Answer from the drawing. Dimensions are ordinates in mm from the lowest x, y and z of the part. Coordinates: 2 decimals unless noted, no trailing zeros. Write each loop counter-clockwise with the first axis right and the second up, starting at its lowest first coordinate (ties: lowest second). Pieces come first, ordered by that corner, then holes.
(1) The part is cut by section A-A, the plane x = 40.5. Determine the outline of the cut face in (y, z).
(2) The part is cut by section C-C, the plane y = 99.5. Determine the outline of the cut face in (x, z).
(3) The part is cut by section D-D, the plane x = 23. Determine the outline of the cut face in (y, z), and give its area (3 significant figures).
(4) Given pin 1 (1.2 mm diameter, centred on y = 154.5, z = 1, fed in from -X); pin 2 (2 mm diameter, centred on x = 26.5, z = 1.5, fed in from +Y), each flat-ended and moving along its own axis, determine where each tip first touches the part or whether it passes through.
(5) The part is cut by section B-B, the plane y = 30.5. Determine the outline of the cut face in (x, z).
(6) Straight lines are drawn through the part: line 1 along X through (y, z) = (16, 3.7); line 2 along Y through (x, z) = (65.5, 3.8); line 3 along Y through (x, z) = (86.5, 2.5). For each, find the intervals that lie inside material, in ascending order.
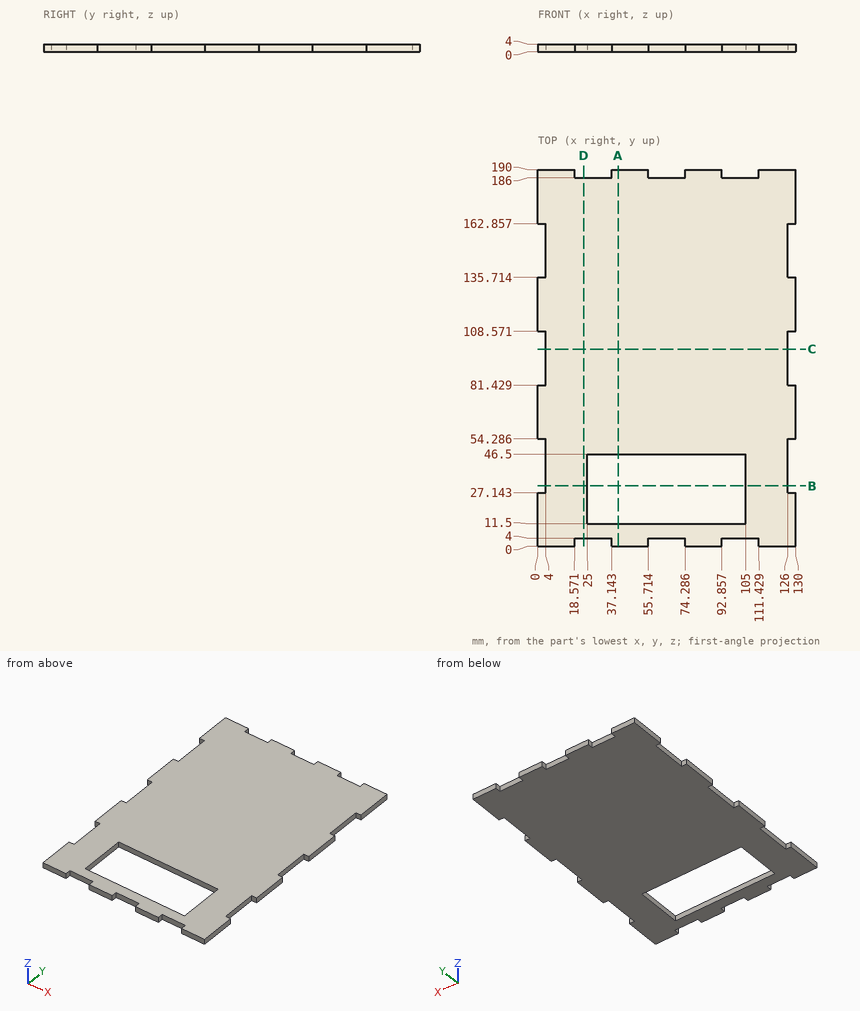
Computed:
1. outline: (0, 0) - (11.5, 0) - (11.5, 4) - (0, 4) - close; (46.5, 0) - (190, 0) - (190, 4) - (46.5, 4) - close
2. outline: (4, 0) - (126, 0) - (126, 4) - (4, 4) - close
3. outline: (4, 0) - (186, 0) - (186, 4) - (4, 4) - close
3. area: 728 mm2
4. pin 1: stops at x = 4
4. pin 2: stops at y = 186
5. outline: (4, 0) - (25, 0) - (25, 4) - (4, 4) - close; (105, 0) - (126, 0) - (126, 4) - (105, 4) - close
6. line 1: x = 0 to 25, 105 to 130
6. line 2: y = 4 to 11.5, 46.5 to 186
6. line 3: y = 0 to 11.5, 46.5 to 190
